Model file for the job. Use its own axes, mm. Face numbers are marked on the shaded views. A direction names the side the tool comes from. Coordinates: 2 decimals unless noted, no trailing zeros. Write each loop counter-clockwise with the first axis right and the second up, starting at its lowest first coordinate (ties: lowest second). Pieces come first, ordered by that corner, then holes.
Q1. Band-saw the part on D-D, the plane z = 6. Write the cut outline in (x, y), plus the area to 3 significant figures.
Q2. Which spindle directions (+Z, -Z, +X, -X, +Y, -Y) get a long thin tool onto all of the face, cutting with end or side? Do the marked faces 1 and 2. Say none if no direction does.
Q3. Drill centre lines: probe 1 along Z at (x, y) = (-6.5, 4.75); probe 2 along Z at (x, y) = (-11.5, 1.9); probe 3 along X at (y, z) = (0.3, 0). Where is each one in solid material? Low to high.
Q4. Pin check, flat tips, straight feed: P1, Ø0.6, axis at x = -11, y = 0.5, coming from the -Z side; P2, Ø0.8, axis at x = -1.5, z = -16, coming from the +Y side; P3, Ø2, axis at x = 1, y = 3.5, coming from the -Z side. Stop position of each tip, or through.
Q5. Band-saw the part on B-B, the plane z = 0. Write the cut outline in (x, y).
Q6. Band-saw the part on C-C, the plane x = -10. Write the cut outline in (y, z).
Q7. Pull direction Z, two halves, no side cores. Call the marked faces 3, 4 and 5: released by +Z, released by -Z, zero draft, split by the parting line, or undercut.
Q8. Band-saw the part on A-A, the plane y = 2.2. State how many separate pieces and enclosed holes the cut face has, plus the area to 3 significant figures.
from build123d import *

# Parameters (mm, degrees)
SKETCH1_R           = 17.5
BOSS_EXTRUDE1_DEPTH = 0.5
SKETCH2_R           = 11.5
CUT_EXTRUDE1_DEPTH  = 0.5
SKETCH3_W           = 15
SKETCH3_H           = 8
CUT_EXTRUDE4_DEPTH  = 2.5
BOSS_EXTRUDE6_DEPTH = 4.5


with BuildPart() as part:
    # Sketch1 → Boss-Extrude1 (new body)
    with BuildSketch(Plane(origin=(0, 0, 0), x_dir=(1, 0, 0), z_dir=(0, 1, 0))):
        with Locations(Location((0, 0, 0), (0, 0, 270))):
            Circle(SKETCH1_R)
    extrude(amount=BOSS_EXTRUDE1_DEPTH)

    # Sketch2 → Cut-Extrude1 (cut)
    with BuildSketch(Plane(origin=(0, 0.5, 0), x_dir=(1, 0, 0), z_dir=(0, 1, 0))):
        with Locations(Location((2, 0, 0), (0, 0, 270))):
            Circle(SKETCH2_R)
    extrude(amount=-CUT_EXTRUDE1_DEPTH, mode=Mode.SUBTRACT)

    # Sketch3 → Cut-Extrude4 (cut)
    with BuildSketch(Plane(origin=(0, 0, 0), x_dir=(1, 0, 0), z_dir=(0, 1, 0))):
        with Locations((-5.5, 0)):
            Rectangle(SKETCH3_W, SKETCH3_H)
    extrude(amount=CUT_EXTRUDE4_DEPTH, mode=Mode.SUBTRACT)

    # Sketch7 → Boss-Extrude6 (add)
    with BuildSketch(Plane(origin=(0, 0.5, 0), x_dir=(1, 0, 0), z_dir=(0, 1, 0))):
        with BuildLine():
            Line((-11.135528726, 13.5), (11.135528726, 13.5))
            ThreePointArc((11.135528726, 13.5), (10.820652744, 13.753671299), (10.5, 14))
            Line((10.5, 14), (-10.5, 14))
            ThreePointArc((-10.5, 14), (-10.820652744, 13.753671299), (-11.135528726, 13.5))
        make_face()
        with BuildLine():
            Line((12.176537068, 12.5), (-12.176537068, 12.5))
            ThreePointArc((-12.176537068, 12.5), (-12.42556977, 12.252480192), (-12.669572012, 12))
            Line((-12.669572012, 12), (12.669572012, 12))
            ThreePointArc((12.669572012, 12), (12.42556977, 12.252480192), (12.176537068, 12.5))
        make_face()
        with BuildLine():
            ThreePointArc((-11.145229996, -13.491992008), (-10.830835088, -13.74565427), (-10.510668849, -13.991992008))
            Line((-10.510668849, -13.991992008), (10.510668849, -13.991992008))
            ThreePointArc((10.510668849, -13.991992008), (10.53333572, -13.974936086), (10.555974914, -13.957843444))
            Line((10.555974914, -13.957843444), (10.555974914, -13.491992008))
            Line((10.555974914, -13.491992008), (-11.145229996, -13.491992008))
        make_face()
        with BuildLine():
            Line((-9.013878189, 15), (9.013878189, 15))
            ThreePointArc((9.013878189, 15), (8.572604405, 15.256488905), (8.124038405, 15.5))
            Line((8.124038405, 15.5), (-8.124038405, 15.5))
            ThreePointArc((-8.124038405, 15.5), (-8.572604405, 15.256488905), (-9.013878189, 15))
        make_face()
        with BuildLine():
            ThreePointArc((-9.027190906, -14.991992008), (-8.586884855, -15.248455938), (-8.139298719, -15.491992008))
            Line((-8.139298719, -15.491992008), (8.139298719, -15.491992008))
            ThreePointArc((8.139298719, -15.491992008), (8.586884855, -15.248455938), (9.027190906, -14.991992008))
            Line((9.027190906, -14.991992008), (-9.027190906, -14.991992008))
        make_face()
        with BuildLine():
            Line((-5.830951895, 16.5), (5.830951895, 16.5))
            ThreePointArc((5.830951895, 16.5), (4.998387844, 16.770990399), (4.153311931, 17))
            Line((4.153311931, 17), (-4.153311931, 17))
            ThreePointArc((-4.153311931, 17), (-4.998387844, 16.770990399), (-5.830951895, 16.5))
        make_face()
        with BuildLine():
            Line((5.853562985, -16.491992008), (-5.853562985, -16.491992008))
            ThreePointArc((-5.853562985, -16.491992008), (-5.025979841, -16.762742217), (-4.185953609, -16.991992008))
            Line((-4.185953609, -16.991992008), (4.185953609, -16.991992008))
            ThreePointArc((4.185953609, -16.991992008), (5.025979841, -16.762742217), (5.853562985, -16.491992008))
        make_face()
        with BuildLine():
            Line((12.669572012, -12), (-12.669572012, -12))
            ThreePointArc((-12.669572012, -12), (-12.42556977, -12.252480192), (-12.176537068, -12.5))
            Line((-12.176537068, -12.5), (12.176537068, -12.5))
            ThreePointArc((12.176537068, -12.5), (12.42556977, -12.252480192), (12.669572012, -12))
        make_face()
    extrude(amount=BOSS_EXTRUDE6_DEPTH)


solid = part.part
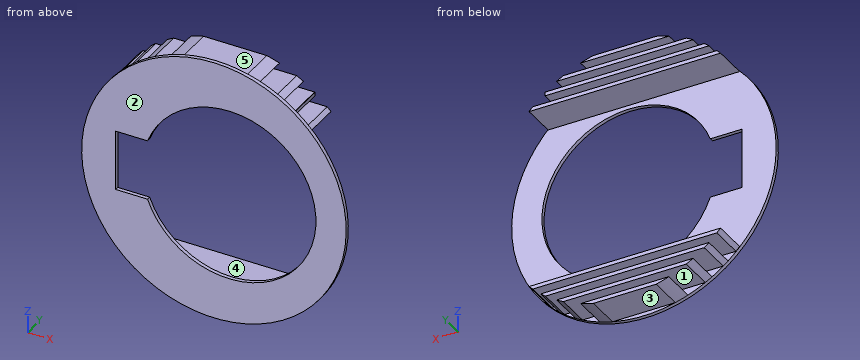
Answer sheet:
1. outline: (-16.44, 0) - (-7.81, 0) - (-7.81, 0.5) - (-16.44, 0.5) - close; (11.81, 0) - (16.44, 0) - (16.44, 0.5) - (11.81, 0.5) - close
1. area: 6.63 mm2
2. face 1: +X, -X, +Y
2. face 2: +Z, -Z, +X, -X, -Y
3. probe 1: z = -15.5 to -15, -14 to -13.5, -12.5 to -12, 12 to 12.5, 13.49 to 13.99, 14.99 to 15.49
3. probe 2: z = -12.5 to -12, 12 to 12.5
3. probe 3: x = -17.5 to -13, 13.5 to 17.5
4. P1: stops at z = -13.85
4. P2: stops at y = 0.5
4. P3: stops at z = -17
5. outline: (-17.5, 0) - (-13, 0) - (-13, 0.5) - (-17.5, 0.5) - close; (13.5, 0) - (17.5, 0) - (17.5, 0.5) - (13.5, 0.5) - close
6. outline: (0, -14.36) - (0.5, -14.36) - (0.5, -14) - (5, -14) - (5, -13.5) - (0.5, -13.5) - (0.5, -12.5) - (5, -12.5) - (5, -12) - (0.5, -12) - (0.5, -4) - (0, -4) - close; (0, 4) - (0.5, 4) - (0.5, 12) - (5, 12) - (5, 12.5) - (0.5, 12.5) - (0.5, 13.49) - (5, 13.49) - (5, 13.99) - (0.5, 13.99) - (0.5, 14.36) - (0, 14.36) - close
7. face 3: released by -Z
7. face 4: undercut
7. face 5: released by +Z
8. separate pieces: 8
8. enclosed holes: 0
8. area: 73.7 mm2
